Can you work these out from the model? Positions are in its coordinate system, mm. A direction names the side the tool comes from. Give positions to 0.01 mm unless a question says otherwise; leave off trailing zeros. Order: outer loops, then holes, each group sorted by start corner. A loop starts at its lowest first (then second) coordinate and runs counter-clockwise, first axis right, second up. Notation, with made-up numbers: M 70,74 L 104,74 A27 cw 104,107 Z; hole C -20,0.25 d11. An arc over 180 degrees is marked long. One line per question, with ' | ' between items. Start each with the question number.
1) If we section it at A-A, the plane x = 0: Please give me the cut outline in (y, z), plus the area to 4 significant figures.
2) If we section it at D-D, the plane z = 72.5: Please give me the cut outline in (x, y).
3) Thinking about a two-plate mould opening in Z: for faces 3 (the cylindrical face through (14.534, 1.479, -41.022)), 4 (the flat face through (-51.5, 2, 50)), 5 (the flat face through (33, 2, -14.997)), 6 (the cylindrical face through (46.906, 1.521, 68.432)), which applies, +Z half, -Z half, draft (parallel to the pull), parting line (faces both ways), or undercut?
4) I'm going to push a flat-ended pin straight in: pin 1 Ø0.9 at (y, z) = (2, -32) entering from -X. Where does the tip first touch, or does it pass through?
5) If we section it at C-C, the plane x = -15: Please give me the cut outline in (y, z), plus the area to 3 significant figures.
6) If we section it at B-B, the plane z = 21.5: Please give me the cut outline in (x, y), plus the area to 3 significant figures.
7) For faces 1 (the flat face through (13.5, 2, 66)), 2 (the flat face through (0, 2, -47.5)), which set-ups out of +Z, -Z, +X, -X, +Y, -Y let a thin tool reach every point of the face, with its end or its side?
8) Please list where these lines run through material, in increasing order: line 1 along X through (y, z) = (0.7, -27.5); line 2 along X through (y, z) = (1.25, 0); line 3 along X through (y, z) = (0.65, 75). Write a range as [from, to].
```python
from build123d import *

# Parameters (mm, degrees)
SKETCH_1_W              = 200
SKETCH_1_H              = 200
EXTRUDE_1_DEPTH         = 3
SKETCH_2_R              = 1.55
CUT_EXTRUDE_2_DEPTH     = 10
CUT_EXTRUDE_3_DEPTH     = 10
SKETCH_6_R              = 1.55
CUT_EXTRUDE_3_1_1_DEPTH = 10
SKETCH_7_R              = 1.55
CUT_EXTRUDE_3_1_2_DEPTH = 113.522220028
CUT_EXTRUDE_21_DEPTH    = 10
CUT_EXTRUDE_6_REACH     = 114.522
SKETCH_10_R             = 3.5


with BuildPart() as part:
    # 草图1 → 凸台-拉伸1 (new body)
    with BuildSketch(Plane(origin=(0, 0, 0), x_dir=(1, 0, 0), z_dir=(0, 1, 0))):
        Rectangle(SKETCH_1_W, SKETCH_1_H)
    extrude(amount=EXTRUDE_1_DEPTH)

    # 草图2 → 切除-拉伸2 (cut)
    with BuildSketch(Plane(origin=(0, 3, 0), x_dir=(1, 0, 0), z_dir=(0, 1, 0))):
        with Locations(Location((29.5, 9.5, 0), (0, 0, 270))):
            Circle(SKETCH_2_R)
        with Locations(Location((21.5, 0, 0), (0, 0, 270))):
            Circle(SKETCH_2_R)
        with Locations(Location((29.5, -9.5, 0), (0, 0, 270))):
            Circle(SKETCH_2_R)
        with Locations(Location((37.5, 0, 0), (0, 0, 270))):
            Circle(SKETCH_2_R)
        with Locations(Location((-29.5, -9.5, 0), (0, 0, 270))):
            Circle(SKETCH_2_R)
        with Locations(Location((-37.5, 0, 0), (0, 0, 270))):
            Circle(SKETCH_2_R)
        with Locations(Location((-21.5, 0, 0), (0, 0, 270))):
            Circle(SKETCH_2_R)
        with Locations(Location((-29.5, 9.5, 0), (0, 0, 270))):
            Circle(SKETCH_2_R)
        with Locations(Location((-15, -32, 0), (0, 0, 270))):
            Circle(SKETCH_2_R)
        with Locations(Location((15, -32, 0), (0, 0, 270))):
            Circle(SKETCH_2_R)
    extrude(amount=-CUT_EXTRUDE_2_DEPTH, mode=Mode.SUBTRACT)

    # 草图5 → 切除-拉伸3 (cut)
    with BuildSketch(Plane(origin=(0, 3, 0), x_dir=(1, 0, 0), z_dir=(0, 1, 0))):
        with BuildLine():
            Line((-51.5, -100), (-51.5, 0))
            Line((-51.5, 0), (-51.5, 0.9969997))
            ThreePointArc((-51.5, 0.9969997), (-47.399494937, 10.896494637), (-37.5, 14.9969997))
            Line((-37.5, 14.9969997), (-29, 14.9969997))
            ThreePointArc((-29, 14.9969997), (-22.636038969, 17.633038669), (-20, 23.9969997))
            Line((-20, 23.9969997), (-20, 24.9949995))
            Line((-20, 24.9949995), (-20, 47.5))
            Line((-20, 47.5), (0, 47.5))
            Line((0, 47.5), (20, 47.5))
            Line((20, 47.5), (20, 24.9949995))
            Line((20, 24.9949995), (20, 23.9969997))
            ThreePointArc((20, 23.9969997), (22.636038969, 17.633038669), (29, 14.9969997))
            Line((29, 14.9969997), (37.5, 14.9969997))
            ThreePointArc((37.5, 14.9969997), (47.399494937, 10.896494637), (51.5, 0.9969997))
            Line((51.5, 0.9969997), (51.5, 0))
            Line((51.5, 0), (51.5, -100))
            Line((51.5, -100), (100, -100))
            Line((100, -100), (100, 100))
            Line((100, 100), (-100, 100))
            Line((-100, 100), (-100, -100))
            Line((-100, -100), (-51.5, -100))
        make_face()
    extrude(amount=-CUT_EXTRUDE_3_DEPTH, mode=Mode.SUBTRACT)

    # 草图6 → φ3.1通孔1 (cut)
    with BuildSketch(Plane.XZ):
        with Locations(Location((-15, -42.5, 0), (0, 0, 270))):
            Circle(SKETCH_6_R)
        with Locations(Location((-15, -27.5, 0), (0, 0, 270))):
            Circle(SKETCH_6_R)
        with Locations(Location((15, -27.5, 0), (0, 0, 90))):
            Circle(SKETCH_6_R)
        with Locations(Location((15, -42.5, 0), (0, 0, 90))):
            Circle(SKETCH_6_R)
    extrude(amount=-CUT_EXTRUDE_3_1_1_DEPTH, mode=Mode.SUBTRACT)

    # 草图7 → φ3.1通孔2 (cut, through all)
    with BuildSketch(Plane(origin=(0, 3, 0), x_dir=(1, 0, 0), z_dir=(0, 1, 0))):
        with Locations(Location((-47.5, -45, 0), (0, 0, 270))):
            Circle(SKETCH_7_R)
        with Locations(Location((-47.5, -67, 0), (0, 0, 270))):
            Circle(SKETCH_7_R)
        with Locations(Location((47.5, -45, 0), (0, 0, 270))):
            Circle(SKETCH_7_R)
        with Locations(Location((47.5, -67, 0), (0, 0, 270))):
            Circle(SKETCH_7_R)
    extrude(amount=-CUT_EXTRUDE_3_1_2_DEPTH, mode=Mode.SUBTRACT)

    # 草图9 → φ21拨单电机孔 (cut)
    with BuildSketch(Plane(origin=(0, 3, 0), x_dir=(1, 0, 0), z_dir=(0, 1, 0))):
        with BuildLine():
            Line((-13.5, -54.75), (-13.5, -76.75))
            ThreePointArc((-13.5, -76.75), (0, -90.25), (13.5, -76.75))
            Line((13.5, -76.75), (13.5, -54.75))
            ThreePointArc((13.5, -54.75), (0, -41.25), (-13.5, -54.75))
        make_face()
    extrude(amount=-CUT_EXTRUDE_21_DEPTH, mode=Mode.SUBTRACT)

    # 草图10 → 切除-拉伸6 (cut, up to next)
    with BuildSketch(Plane.XZ, mode=Mode.PRIVATE) as cut_extrude_6_sk1:
        with Locations(Location((-31.5, 21.5, 0), (0, 0, 270))):
            Circle(SKETCH_10_R)
    cut_extrude_6_tool1 = extrude(cut_extrude_6_sk1.sketch, amount=-CUT_EXTRUDE_6_REACH, mode=Mode.PRIVATE) & part.part
    # 草图10 → 切除-拉伸6 (cut, up to next)
    with BuildSketch(Plane.XZ, mode=Mode.PRIVATE) as cut_extrude_6_sk2:
        with Locations(Location((31.5, 21.5, 0), (0, 0, 270))):
            Circle(SKETCH_10_R)
    cut_extrude_6_tool2 = extrude(cut_extrude_6_sk2.sketch, amount=-CUT_EXTRUDE_6_REACH, mode=Mode.PRIVATE) & part.part
    add(cut_extrude_6_tool1.solids().sort_by_distance((-31.5, 0, 21.5))[0], mode=Mode.SUBTRACT)
    add(cut_extrude_6_tool2.solids().sort_by_distance((31.5, 0, 21.5))[0], mode=Mode.SUBTRACT)


solid = part.part
```
Results found:
1) outline: M 0,-47.5 L 3,-47.5 L 3,41.25 L 0,41.25 Z; M 0,90.25 L 3,90.25 L 3,100 L 0,100 Z | area: 295.5 mm²
2) outline: M -51.5,0 L -13.5,0 L -13.5,3 L -51.5,3 Z; M 13.5,0 L 51.5,0 L 51.5,3 L 13.5,3 Z
3) face 3: undercut | face 4: draft | face 5: -Z half | face 6: undercut
4) pin 1: stops at x = -20
5) outline: M 0,-47.5 L 3,-47.5 L 3,-44.05 L 0,-44.05 Z; M 0,-40.95 L 3,-40.95 L 3,-29.05 L 0,-29.05 Z; M 0,-25.95 L 3,-25.95 L 3,30.45 L 0,30.45 Z; M 0,33.55 L 3,33.55 L 3,100 L 0,100 Z | area: 415 mm²
6) outline: M -51.5,0 L -35,0 L -35,3 L -51.5,3 Z; M -28,0 L 28,0 L 28,3 L -28,3 Z; M 35,0 L 51.5,0 L 51.5,3 L 35,3 Z | area: 267 mm²
7) face 1: +Y, -Y | face 2: -Z, +X, -X, +Y, -Y
8) line 1: x = [-20, -16.55], [-13.45, 13.45], [16.55, 20] | line 2: x = [-51.5, -39.05], [-35.95, -23.05], [-19.95, 19.95], [23.05, 35.95], [39.05, 51.5] | line 3: x = [-51.5, -13.5], [13.5, 51.5]
